Verification items for this drawing (mm, ordinates from the low corner). A direction names the side the tool comes from. Round coordinates to 2 decimals unless told otherwise and drop trailing zeros. Order: outer loops, then holes, each group sorted by start corner. A loop starts at its lowest first (then second) coordinate and runs counter-clockwise, first axis right, second up. Notation, with made-up numbers: M 49.25,35.25 L 62.25,35.25 A14 cw 62.25,40.25 Z; hole C 43,24.5 d9. An arc over 180 degrees is marked long. Use CSV: the item, a comma, the result in double quotes. Start each with the question number.
Q1. Gauge pin test, flat ends, axial feed: pin 1 Ø6 at (x, z) = (27, 23.5) entering from -Y; pin 2 Ø12 at (y, z) = (97, 5) entering from +X; pin 3 Ø1.5 at (y, z) = (119.5, 6) entering from -X. Record the tip position at first contact, or that the pin passes through.
Q2. Sectioned sample at A-A (y = 75). Enter the section's corners in (x, z).
Q3. Scan lines: line 1 (Y direction, x = 75, z = 4.25); line 2 (Z direction, x = 63, y = 123); line 3 (X direction, y = 63, z = 3) (1 decimal). Record each from-to range of solid material in increasing order.
Q4. Sectioned sample at C-C (z = 24.5). State how many separate pieces and enclosed holes the cut face has.
Q5. Set-up check for the marked faces 1, 2, 3 and 4: record each of +Z, -Z, +X, -X, +Y, -Y from which the full face is reachable in a straight line by a thin tool's end or side.
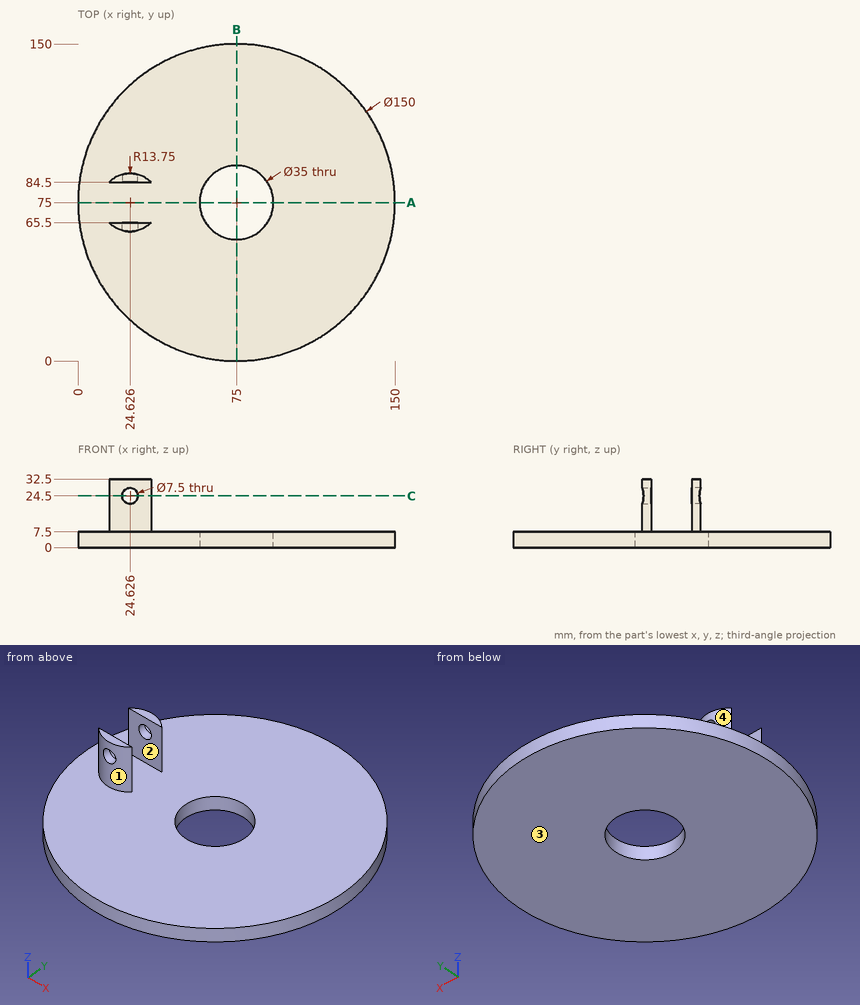
Verdict:
1,pin 1,"stops at y = 61.28"
1,pin 2,"stops at x = 148.27"
1,pin 3,"stops at x = 14.08"
2,outline,"M 0,0 L 57.5,0 L 57.5,7.5 L 0,7.5 Z; M 92.5,0 L 150,0 L 150,7.5 L 92.5,7.5 Z"
3,line 1,"y = 0 to 57.5, 92.5 to 150"
3,line 2,"z = 0 to 7.5"
3,line 3,"x = 1 to 62.3, 87.7 to 149"
4,separate pieces,"4"
4,enclosed holes,"0"
5,face 1,"+Z, -Y"
5,face 2,"+Z, +X, -X"
5,face 3,"-Z, +X, -X, +Y, -Y"
5,face 4,"+Z, +Y"
